```python
from build123d import *

# Parameters (mm, degrees)
SKETCH_1_R               = 35
EXTRUDE_1_DEPTH          = 9
CUT_EXTRUDE_1_DEPTH      = 51.309044912
CUT_EXTRUDE_1_DEPTH_BACK = 51.309044912
CUT_EXTRUDE_2_DEPTH      = 51.309044912
CUT_EXTRUDE_2_DEPTH_BACK = 51.309044912
SKETCH_3_R               = 3.5
SKETCH_3_R_2             = 6.5
SKETCH_4_W               = 1
SKETCH_4_H               = 6


with BuildPart() as part:
    # 스케치1 → 보스-돌출1 (new body)
    with BuildSketch(Plane(origin=(0, 0, 0), x_dir=(1, 0, 0), z_dir=(0, 1, 0))):
        with Locations(Location((0, 0, 0), (0, 0, 270))):
            Circle(SKETCH_1_R)
    extrude(amount=EXTRUDE_1_DEPTH)

    # 스케치2 → 컷-돌출1 (cut, two sides: drawn at the far end of the back side and taken through both)
    with BuildSketch(Plane(origin=(0, 9, 0), x_dir=(1, 0, 0), z_dir=(0, 1, 0)).offset(-CUT_EXTRUDE_1_DEPTH_BACK)):
        with BuildLine():
            Line((-1.658312395, 2.5), (1.658312395, 2.5))
            ThreePointArc((1.658312395, 2.5), (0, -3), (-1.658312395, 2.5))
        make_face()
    extrude(amount=CUT_EXTRUDE_1_DEPTH + CUT_EXTRUDE_1_DEPTH_BACK, mode=Mode.SUBTRACT)

    # 스케치3 → 컷-돌출2 (cut, two sides: drawn at the far end of the back side and taken through both)
    with BuildSketch(Plane(origin=(0, 9, 0), x_dir=(1, 0, 0), z_dir=(0, 1, 0)).offset(-CUT_EXTRUDE_2_DEPTH_BACK)):
        with Locations(Location((8.485281374, -8.485281374, 0), (0, 0, 270))):
            Circle(SKETCH_3_R)
        with Locations(Location((8.419035512, -20.325349715, 0), (0, 0, 270))):
            Circle(SKETCH_3_R_2)
        with Locations(Location((-8.419035512, -20.325349715, 0), (0, 0, 270))):
            Circle(SKETCH_3_R_2)
        with Locations(Location((0, -12, 0), (0, 0, 270))):
            Circle(SKETCH_3_R)
        with Locations(Location((-20.325349715, -8.419035512, 0), (0, 0, 270))):
            Circle(SKETCH_3_R_2)
        with Locations(Location((-8.485281374, -8.485281374, 0), (0, 0, 270))):
            Circle(SKETCH_3_R)
        with Locations(Location((-20.325349715, 8.419035512, 0), (0, 0, 270))):
            Circle(SKETCH_3_R_2)
        with Locations(Location((-12, 0, 0), (0, 0, 270))):
            Circle(SKETCH_3_R)
        with Locations(Location((-8.419035512, 20.325349715, 0), (0, 0, 270))):
            Circle(SKETCH_3_R_2)
        with Locations(Location((-8.485281374, 8.485281374, 0), (0, 0, 270))):
            Circle(SKETCH_3_R)
        with Locations(Location((8.419035512, 20.325349715, 0), (0, 0, 270))):
            Circle(SKETCH_3_R_2)
        with Locations(Location((0, 12, 0), (0, 0, 270))):
            Circle(SKETCH_3_R)
        with Locations(Location((20.325349715, 8.419035512, 0), (0, 0, 270))):
            Circle(SKETCH_3_R_2)
        with Locations(Location((8.485281374, 8.485281374, 0), (0, 0, 270))):
            Circle(SKETCH_3_R)
        with Locations(Location((20.325349715, -8.419035512, 0), (0, 0, 270))):
            Circle(SKETCH_3_R_2)
        with Locations(Location((12, 0, 0), (0, 0, 270))):
            Circle(SKETCH_3_R)
    extrude(amount=CUT_EXTRUDE_2_DEPTH + CUT_EXTRUDE_2_DEPTH_BACK, mode=Mode.SUBTRACT)

    # 스케치4 → 컷-회전1 (revolve, cut)
    with BuildSketch(Plane(origin=(0, 0, 0), x_dir=(0, 0, -1), z_dir=(1, 0, 0)), mode=Mode.PRIVATE) as cut_revolve_1_sk:
        with Locations((35, 4.5)):
            Rectangle(SKETCH_4_W, SKETCH_4_H)
    revolve(cut_revolve_1_sk.sketch.rotate(Axis((0, 9, 0), (0, -1, 0)), 180), axis=Axis((0, 9, 0), (0, -1, 0)), mode=Mode.SUBTRACT)


solid = part.part
```
CAD build for the part. Positions are in the model's coordinates, mm. A direction names the side the tool comes from. Coordinates: 2 decimals unless noted, no trailing zeros. Write each loop counter-clockwise with the first axis right and the second up, starting at its lowest first coordinate (ties: lowest second). Pieces come first, ordered by that corner, then holes. Notation, with made-up numbers: (-11, 24.5) -> (27, 24.5) arc R18 cw to (27, 49.5) -> close; hole circle Ø2 at (35, -3.75). An arc over 180 degrees is marked (long way). Return JSON: item names as keys, results as strings. Group by question number.
Q1. Flat gauge pins, fed straight in: pin 1 (8 mm diameter, centred on x = -8.49, z = -8.49, fed in from -Y); pin 2 (1.5 mm diameter, centred on y = 5.5, z = 25, fed in from -X); pin 3 (2 mm diameter, centred on y = 4.5, z = -24.5, fed in from +X); pin 4 (2 mm diameter, centred on x = -16.5, y = 7, fed in from +Z). Where does each tip first touch, or does it go through?
Q2. Cut at B-B, the plane x = 0. Give the cut face in (y, z).
Q3. Cut at C-C, the plane z = 10.5. State how many separate pieces and enclosed holes the cut face has, then the cut area to 3 significant figures.
Q4. Drill centre lines: line 1 (Z direction, x = -4, y = 5.5); line 2 (Z direction, x = 26, y = 7); line 3 (X direction, y = 7, z = 25). Where is each one in solid material? Low to high.
Q5. Pull direction Z, two halves, no side cores. Call faces 1 (the face through (-7, 9, 0)), 2 (the face through (-21, 1, -28)), 3 (the face through (16.4, 4.4, -13.6)): released by +Z, released by -Z, zero draft, split by the parting line, or undercut.
Q6. Cut at A-A, the plane z = 0. Give the cut face in (x, y), then the cut area to 3 significant figures.
Q7. Which spindle directions (+Z, -Z, +X, -X, +Y, -Y) get a long thin tool onto all of the face, cutting with end or side? Do faces 4 (the face through (-7, 0, 0)), 5 (the face through (-1.517, 4.542, -34.467)), 6 (the face through (0, 4, -2.5)). Say none if no direction does.
Returned:
{
 "1": {"pin 1": "stops at y = 0", "pin 2": "stops at x = -24.54", "pin 3": "stops at x = 25.26", "pin 4": "stops at z = 31.31"},
 "2": {"outline": "(0, -35) -> (1.5, -35) -> (1.5, -34.5) -> (7.5, -34.5) -> (7.5, -35) -> (9, -35) -> (9, -15.5) -> (0, -15.5) -> close; (0, -8.5) -> (9, -8.5) -> (9, -2.5) -> (0, -2.5) -> close; (0, 3) -> (9, 3) -> (9, 8.5) -> (0, 8.5) -> close; (0, 15.5) -> (9, 15.5) -> (9, 35) -> (7.5, 35) -> (7.5, 34.5) -> (1.5, 34.5) -> (1.5, 35) -> (0, 35) -> close"},
 "3": {"separate pieces": "6", "enclosed holes": "0", "area": "213 mm2"},
 "4": {"line 1": "z = -34.27 to -25.09, -15.56 to 15.56, 25.09 to 34.27", "line 2": "z = -22.68 to -11.59, -5.25 to 5.25, 11.59 to 22.68", "line 3": "x = -23.77 to -12.94, -3.9 to 3.9, 12.94 to 23.77"},
 "5": {"face 1": "zero draft", "face 2": "split by the parting line", "face 3": "undercut"},
 "6": {"outline": "(-35, 0) -> (-15.5, 0) -> (-15.5, 9) -> (-35, 9) -> (-35, 7.5) -> (-34.5, 7.5) -> (-34.5, 1.5) -> (-35, 1.5) -> close; (-8.5, 0) -> (-3, 0) -> (-3, 9) -> (-8.5, 9) -> close; (3, 0) -> (8.5, 0) -> (8.5, 9) -> (3, 9) -> close; (15.5, 0) -> (35, 0) -> (35, 1.5) -> (34.5, 1.5) -> (34.5, 7.5) -> (35, 7.5) -> (35, 9) -> (15.5, 9) -> close", "area": "444 mm2"},
 "7": {"face 4": "+Z, -Z, +X, -X, -Y", "face 5": "none", "face 6": "+Y, -Y"}
}
